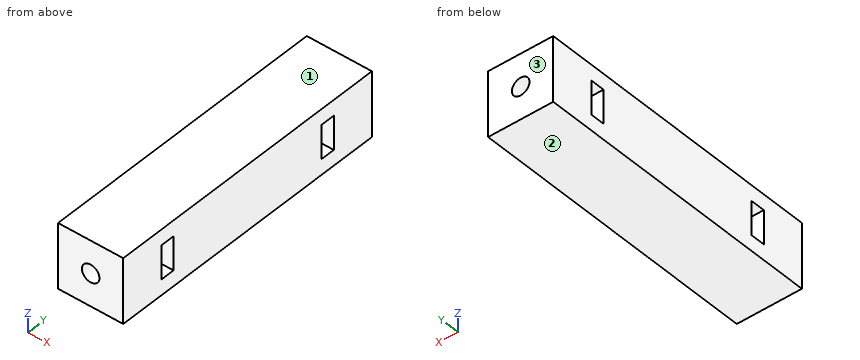
Autodesk Inventor part; units mm, degrees
ref_plane "YZ Plane" through (0, 0, 0) normal (1, 0, 0) x (0, 1, 0)
ref_plane "XZ Plane" through (0, 0, 0) normal (0, 1, 0) x (-1, 0, 0)
ref_plane "XY Plane" through (0, 0, 0) normal (0, 0, 1) x (1, 0, 0)
sketch "스케치1" plane through (0, 0, 0) normal (0, 1, 0) x (-1, 0, 0)
  line L0 (-5, 5) -> (5, 5)
  line L1 (5, 5) -> (5, -5)
  line L2 (5, -5) -> (-5, -5)
  line L3 (-5, -5) -> (-5, 5)
  line L4 (-5, 5) -> (5, -5) construction
  line L5 (5, 5) -> (-5, -5) construction
  circle A0 centre (0, 0) radius 1.35
  dimension "d0" = 10
  dimension "d1" = 10
  dimension "d2" = 2.7
extrude "돌출1" add sketch "스케치1" along normal blind 45 contours L0 L1 L2 L3 | A0
sketch "스케치2" plane through (0, 0, 0) normal (0, -1, 0) x (1, 0, 0)
  circle A0 centre (0, 0) radius 1.35
  dimension "d5" = 2.7
extrude "돌출2" cut sketch "스케치2" against normal blind 16
sketch "스케치3" plane through (0, 45, 0) normal (0, 1, 0) x (1, 0, 0)
  circle A0 centre (0, 0) radius 1.35
  dimension "d8" = 2.7
extrude "돌출3" cut sketch "스케치3" against normal blind 16
sketch "스케치4" plane through (5, 0, 5) normal (1, 0, 0) x (0, 0, -1)
  line L0 (0, 45) -> (10, 45)
  line L1 (10, 45) -> (0, 45)
  line L2 (3.65, 45) -> (6.35, 45)
  line L3 (3.65, 29) -> (6.35, 29)
  line L4 (3.65, 45) -> (6.35, 45)
  line L5 (10, 45) -> (0, 45)
  line L6 (0, 45) -> (10, 45)
  line L7 (3.65, 29) -> (6.35, 29)
  line L8 (3.65, 29) -> (6.35, 29)
  line L9 (3.65, 45) -> (6.35, 45)
  line L10 (10, 0) -> (0, 0)
  line L11 (0, 0) -> (10, 0)
  line L12 (6.35, 0) -> (3.65, 0)
  line L13 (6.35, 16) -> (3.65, 16)
  line L14 (6.35, 0) -> (3.65, 0)
  line L15 (0, 0) -> (10, 0)
  line L16 (10, 0) -> (0, 0)
  line L17 (6.35, 16) -> (3.65, 16)
  line L18 (6.35, 16) -> (3.65, 16)
  line L19 (6.35, 0) -> (3.65, 0)
  line L20 (10, 0) -> (10, 45)
  line L21 (0, 0) -> (0, 45)
  line L22 (0, 0) -> (0, 45)
  line L23 (10, 0) -> (10, 45)
  line L24 (10, 0) -> (10, 45)
  line L25 (10, 0) -> (10, 45)
  line L26 (10, 0) -> (0, 0)
  line L27 (0, 0) -> (0, 45)
  line L28 (10, 45) -> (0, 45)
  line L29 (10, 0) -> (10, 45)
  line L30 (0, 0) -> (0, 45)
  line L31 (0, 0) -> (0, 45)
  line L32 (0, 0) -> (10, 0)
  line L33 (10, 0) -> (10, 45)
  line L34 (0, 45) -> (10, 45)
  line L35 (0, 0) -> (0, 45)
  line L36 (3.65, 45) -> (3.65, 29)
  line L37 (6.35, 45) -> (6.35, 29)
  line L38 (3.65, 0) -> (3.65, 16)
  line L39 (6.35, 0) -> (6.35, 16)
  line L40 (2.4, 38.1) -> (7.6, 38.1)
  line L41 (7.6, 38.1) -> (7.6, 35.9)
  line L42 (7.6, 35.9) -> (2.4, 35.9)
  line L43 (2.4, 35.9) -> (2.4, 38.1)
  line L44 (2.4, 38.1) -> (7.6, 35.9) construction
  line L45 (7.6, 38.1) -> (2.4, 35.9) construction
  line L46 (2.4, 6.9) -> (7.6, 6.9)
  line L47 (7.6, 6.9) -> (7.6, 9.1)
  line L48 (7.6, 9.1) -> (2.4, 9.1)
  line L49 (2.4, 9.1) -> (2.4, 6.9)
  line L50 (2.4, 6.9) -> (7.6, 9.1) construction
  line L51 (7.6, 6.9) -> (2.4, 9.1) construction
  point P0 (5, 0)
  point P1 (5, 37)
  point P2 (5, 8)
  dimension "d11" = 5.2
  dimension "d12" = 2.2
  dimension "d13" = 5.2
  dimension "d14" = 2.2
extrude "돌출4" cut sketch "스케치4" against normal blind 16 contours L40 L37 L42 L36 | L36 L42 L43 L40 | L40 L41 L42 L37 | L46 L49 L48 L38 | L38 L48 L39 L46 | L39 L48 L47 L46
properties part number "frame_head2" material "PMMA 플라스틱"
Design review of the part built by this model. Coordinates are the model's own, in mm. Face numbers are marked on the shaded views. Give positions to 0.01 mm unless a question says otherwise; leave off trailing zeros. Loops run counter-clockwise (first coordinate to the right, second up) from the corner with the lowest first, then second, coordinate; pieces in that order, holes last. Notation, with made-up numbers: M 27,86 L 86,86 A15 ccw 86,92 Z; hole C -26,-32 d6. An arc over 180 degrees is marked long. One line per question, with ' | ' between items. Start each with the question number.
1. Add section B-B (x = 2.25). Write out the cut boundary in (y, z).
2. Add section D-D (y = 35). Write out the cut boundary in (x, z), plus the area to 3 significant figures.
3. Add section C-C (x = 0). Write out the cut boundary in (y, z).
4. Add section A-A (z = 0). Write out the cut boundary in (x, y), plus the area to 3 significant figures.
5. To check wall thickness, follow L1, parallel to Y at x = -1.5, z = 1; L2, parallel to Z at x = 0, y = 7; L3, parallel to Z at x = 0, y = 3. State the ranges of each line that lie inside material, in increasing order.
6. Insertion check: P1, Ø2.5, axis at x = 0, z = 0, coming from the +Y side. The pin has a flat end and moves straight along its axis. Give the tip position at first contact, or say it passes through.
7. The part is to be moulded in two halves that separate along Z. For the marked faces 1, 2 and 3, say which applies: released by +Z, released by -Z, zero draft, split by the parting line, or undercut.
Worked out:
1) outline: M 0,-5 L 45,-5 L 45,5 L 0,5 Z; hole M 6.9,-2.6 L 9.1,-2.6 L 9.1,2.6 L 6.9,2.6 Z; hole M 35.9,-2.6 L 38.1,-2.6 L 38.1,2.6 L 35.9,2.6 Z
2) outline: M -5,-5 L 5,-5 L 5,5 L -5,5 Z; hole C 0,0 d2.7 | area: 94.3 mm²
3) outline: M 0,-5 L 45,-5 L 45,-1.35 L 38.1,-1.35 L 38.1,-2.6 L 35.9,-2.6 L 35.9,-1.35 L 29,-1.35 L 29,1.35 L 35.9,1.35 L 35.9,2.6 L 38.1,2.6 L 38.1,1.35 L 45,1.35 L 45,5 L 0,5 L 0,1.35 L 6.9,1.35 L 6.9,2.6 L 9.1,2.6 L 9.1,1.35 L 16,1.35 L 16,-1.35 L 9.1,-1.35 L 9.1,-2.6 L 6.9,-2.6 L 6.9,-1.35 L 0,-1.35 Z
4) outline: M -5,0 L -1.35,0 L -1.35,6.9 L -5,6.9 Z; M -5,9.1 L -1.35,9.1 L -1.35,16 L 1.35,16 L 1.35,9.1 L 5,9.1 L 5,35.9 L 1.35,35.9 L 1.35,29 L -1.35,29 L -1.35,35.9 L -5,35.9 Z; M -5,38.1 L -1.35,38.1 L -1.35,45 L -5,45 Z; M 1.35,0 L 5,0 L 5,6.9 L 1.35,6.9 Z; M 1.35,38.1 L 5,38.1 L 5,45 L 1.35,45 Z | area: 331 mm²
5) L1: y = 0 to 6.9, 9.1 to 35.9, 38.1 to 45 | L2: z = -5 to -2.6, 2.6 to 5 | L3: z = -5 to -1.35, 1.35 to 5
6) P1: stops at y = 29
7) face 1: released by +Z | face 2: released by -Z | face 3: zero draft
